Input: part model. Units: mm. Frame: model coordinates. A direction names the side the tool comes from. Coordinates: 2 decimals unless noted, no trailing zeros. Loops run counter-clockwise (first coordinate to the right, second up) from the corner with the lowest first, then second, coordinate; pieces in that order, holes last. Notation, with made-up numbers: (-3.5, 54.25) - (20.5, 54.25) arc R10 ccw to (20.5, 61.25) - close; hole circle Ø5 at (-21, 52). An arc over 180 degrees is marked (long way). Use a Markdown table: item, result. Add a question column.
1. Contact query for flat-ended pins moving along their axis: P1, Ø20.5, axis at x = -3.5, y = 8.5, coming from the -Z side; P2, Ø10.5, axis at x = 4.5, z = -12.5, coming from the -Y side. Output: stop coordinate, or through.
2. Access query for faces 1 (the face through (-1, 51.308, -12)), 2 (the face through (0, 25.908, -18)). Directions: +Z, -Z, +X, -X, +Y, -Y. A direction counts if a zero-diameter tool reaches every point of the face in a straight line with its end or side. Return the directions, or none.
3. Ray query, L1, parallel to X at y = 33.5, z = -24; L2, parallel to X at y = 31.5, z = -30.5; L3, parallel to Z at x = -18.5, y = 25. Return the intervals inside material, ascending. Write a range as [from, to].
4. Section query C-C on y = 17.5. Return the cut outline in (x, z).
5. Section query B-B on y = 40. Return the cut outline in (x, z), then the cut area to 3 significant figures.
6. Section query A-A on z = -17.78. State how many separate pieces and enclosed holes the cut face has, then the cut area to 3 significant figures.
7. Draft query along Z for faces 3 (the face through (26.18, 41.61, -31.25)), 4 (the face through (-1, 0, 6)), 5 (the face through (-1, 39, -35.814)), 6 (the face through (-1, 25, 12.7)). Return one class per face: released by +Z, released by -Z, zero draft, split by the parting line, or undercut.
```python
from build123d import *

# Parameters (mm, degrees)
SKETCH1_W           = 76.454
SKETCH1_H           = 12.7
BOSS_EXTRUDE1_DEPTH = 51.308
SKETCH2_W           = 76.454
SKETCH2_H           = 35.814
BOSS_EXTRUDE2_DEPTH = 25.4
SKETCH3_R           = 17.145
SKETCH4_R           = 13.97
SKETCH3_3_R         = 17.145
SKETCH4_3_R         = 13.97


with BuildPart() as part:
    # Sketch1 → Boss-Extrude1 (new body)
    with BuildSketch(Plane(origin=(0, 0, 0), x_dir=(1, 0, 0), z_dir=(0, 1, 0))):
        with Locations((0, -6.35)):
            Rectangle(SKETCH1_W, SKETCH1_H)
    extrude(amount=BOSS_EXTRUDE1_DEPTH)

    # Sketch2 → Boss-Extrude2 (add)
    with BuildSketch(Plane(origin=(0, 51.308, 0), x_dir=(1, 0, 0), z_dir=(0, 1, 0))):
        with Locations((0, 17.907)):
            Rectangle(SKETCH2_W, SKETCH2_H)
    extrude(amount=-BOSS_EXTRUDE2_DEPTH)

    # Sketch3 → Cut-Loft2 section 0
    with BuildSketch(Plane.XZ.offset(-25.908)):
        with Locations((19.177, -17.78)):
            Circle(SKETCH3_R)
    # Sketch4 → Cut-Loft2 section 1
    with BuildSketch(Plane(origin=(0, 51.308, 0), x_dir=(1, 0, 0), z_dir=(0, 1, 0))):
        with Locations((19.177, 17.78)):
            Circle(SKETCH4_R)
    loft(mode=Mode.SUBTRACT)

    # Sketch3<3> → Cut-Loft3 section 0
    with BuildSketch(Plane.XZ.offset(-25.908)):
        with Locations((-19.177, -17.78)):
            Circle(SKETCH3_3_R)
    # Sketch4<3> → Cut-Loft3 section 1
    with BuildSketch(Plane(origin=(0, 51.308, 0), x_dir=(1, 0, 0), z_dir=(0, 1, 0))):
        with Locations((-19.177, 17.78)):
            Circle(SKETCH4_3_R)
    loft(mode=Mode.SUBTRACT)


solid = part.part
```
Resolved:
| question | item | result |
|---|---|---|
| 1 | P1 | z = 0 |
| 1 | P2 | y = 25.91 |
| 2 | face 1 | +Z, -Z, +X, -X, +Y |
| 2 | face 2 | -Z, +X, -X, -Y |
| 3 | L1 | [-38.23, -34.13], [-4.22, 4.22], [34.13, 38.23] |
| 3 | L2 | [-38.23, -29.6], [-8.75, 8.75], [29.6, 38.23] |
| 3 | L3 | [0, 12.7] |
| 4 | outline | (-38.23, 0) - (38.23, 0) - (38.23, 12.7) - (-38.23, 12.7) - close |
| 5 | outline | (-38.23, -35.81) - (38.23, -35.81) - (38.23, 12.7) - (-38.23, 12.7) - close; hole circle Ø30.77 at (-19.18, -17.78); hole circle Ø30.77 at (19.18, -17.78) |
| 5 | area | 2,220 mm² |
| 6 | separate pieces | 3 |
| 6 | enclosed holes | 0 |
| 6 | area | 361 mm² |
| 7 | face 3 | undercut |
| 7 | face 4 | zero draft |
| 7 | face 5 | released by -Z |
| 7 | face 6 | released by +Z |
